from build123d import *

# Parameters (mm, degrees)
SALIENTE_EXTRUIR1_DEPTH = 2
SALIENTE_EXTRUIR2_DEPTH = 2
SALIENTE_EXTRUIR3_DEPTH = 2
CROQUIS5_W              = 22
CROQUIS5_H              = 2
SALIENTE_EXTRUIR4_DEPTH = 17
CROQUIS6_W              = 26
CROQUIS6_H              = 2
SALIENTE_EXTRUIR5_DEPTH = 3
CROQUIS7_W              = 9.109165418
CROQUIS7_H              = 2
CROQUIS7_W_2            = 9.958756631
SALIENTE_EXTRUIR6_DEPTH = 20
CHAFL_N1_SIZE           = 1
CHAFL_N2_SIZE           = 1
CHAFL_N2_SIZE_2         = 0.713515305
CROQUIS8_R              = 8
SALIENTE_EXTRUIR7_DEPTH = 9


with BuildPart() as part:
    # Croquis1 → Saliente-Extruir1 (new body)
    with BuildSketch(Plane.XY):
        Polygon((-2, 23.6), (-2, 20.4), (-2, -5.284781413), (24, -5.284781413), (24, 20.4), (24, 23.6), align=None)
    extrude(amount=SALIENTE_EXTRUIR1_DEPTH)

    # Croquis2 → Saliente-Extruir2 (add)
    with BuildSketch(Plane(origin=(24, 0, 0), x_dir=(0, 0, -1), z_dir=(1, 0, 0))):
        Polygon((0, 23.6), (37.896029649, 23.6), (0, -5.284781413), align=None)
    extrude(amount=-SALIENTE_EXTRUIR2_DEPTH)

    # Croquis4 → Saliente-Extruir3 (add)
    with BuildSketch(Plane.ZY.offset(2)):
        with BuildLine():
            Line((-37.896029649, 23.6), (0, 23.6))
            Line((0, 23.6), (0, -5.284781413))
            Line((0, -5.284781413), (-9.534216457, 1.982305954))
            ThreePointArc((-9.534216457, 1.982305954), (-4.573867025, 12.209468647), (-13.454047634, 19.304700538))
            Line((-13.454047634, 19.304700538), (-32.260716249, 19.304700538))
            Line((-32.260716249, 19.304700538), (-37.896029649, 23.6))
        make_face()
    extrude(amount=-SALIENTE_EXTRUIR3_DEPTH)

    # Croquis5 → Saliente-Extruir4 (add)
    with BuildSketch(Plane(origin=(0, 0, 0), x_dir=(-1, 0, 0), z_dir=(0, 0, -1))):
        with Locations((-11, 22.6)):
            Rectangle(CROQUIS5_W, CROQUIS5_H)
    extrude(amount=SALIENTE_EXTRUIR4_DEPTH)

    # Croquis6 → Saliente-Extruir5 (add)
    with BuildSketch(Plane(origin=(0, 0, 0), x_dir=(-1, 0, 0), z_dir=(0, 0, -1))):
        with Locations((-11, -4.284781413)):
            Rectangle(CROQUIS6_W, CROQUIS6_H)
    extrude(amount=SALIENTE_EXTRUIR5_DEPTH)

    # Croquis7 → Saliente-Extruir6 (add)
    with BuildSketch(Plane(origin=(0, 0, -17), x_dir=(-1, 0, 0), z_dir=(0, 0, -1))):
        with Locations((-4.554582709, 22.6)):
            Rectangle(CROQUIS7_W, CROQUIS7_H)
        with Locations((-17.020621685, 22.6)):
            Rectangle(CROQUIS7_W_2, CROQUIS7_H)
    extrude(amount=SALIENTE_EXTRUIR6_DEPTH)

    # Chaflán1
    chafl_n1_edges = [part.edges().sort_by_distance(p)[0] for p in [
        (17.020621684, 21.6, -37),
        (4.554582709, 21.6, -37),
    ]]
    chamfer(chafl_n1_edges, length=CHAFL_N1_SIZE)

    # Chaflán2
    # the kernel refuses this chamfer: 1, 0.713515305 mm, written as the material it takes off along each edge
    with BuildSketch(Plane(origin=(26.571682988, 23.6, -37.896029649), x_dir=(0, 0, 1), z_dir=(-1, 0, 0))) as chafl_n2_piece_1:
        Polygon((CHAFL_N2_SIZE, 0), (CHAFL_N2_SIZE_2 * 0.79531418588, -CHAFL_N2_SIZE_2 * 0.606197446726), (0, 0), align=None)
    extrude(amount=7.143365976, mode=Mode.SUBTRACT)
    # the kernel refuses this chamfer: 1, 0.713515305 mm, written as the material it takes off along each edge
    with BuildSketch(Plane(origin=(22, 23.6, -37), x_dir=(0, 0, 1), z_dir=(-1, 0, 0))) as chafl_n2_2_piece_1_section:
        Polygon((CHAFL_N2_SIZE, 0), (0, -CHAFL_N2_SIZE), (0, 0), align=None)
    chafl_n2_2_piece_1 = extrude(amount=12.530439619, mode=Mode.PRIVATE)
    chafl_n2_2_piece_1 = split(chafl_n2_2_piece_1, bisect_by=Plane(origin=(22, 23.548014824, -36.948014824), z_dir=(-1.533293416683386e-15, 0.7071067811865533, -0.7071067811865418)), keep=Keep.TOP, mode=Mode.PRIVATE)
    add(chafl_n2_2_piece_1, mode=Mode.SUBTRACT)
    # the kernel refuses this chamfer: 1, 0.713515305 mm, written as the material it takes off along each edge
    with BuildSketch(Plane(origin=(-4.571682988, 23.6, -37.896029649), x_dir=(0, -0.6061974471264424, 0.7953141864052119), z_dir=(1, 0, 0))) as chafl_n2_3_piece_1:
        Polygon((CHAFL_N2_SIZE, 0), (CHAFL_N2_SIZE_2 * 0.79531418588, -CHAFL_N2_SIZE_2 * 0.606197446726), (0, 0), align=None)
    extrude(amount=7.143365976, mode=Mode.SUBTRACT)

    # Croquis8 → Saliente-Extruir7 (add)
    with BuildSketch(Plane.XY.offset(2)):
        with Locations((11, 9.157609293)):
            Circle(CROQUIS8_R)
    extrude(amount=SALIENTE_EXTRUIR7_DEPTH)


solid = part.part
Read the model definition and answer for the solid it produces. Units are mm, in the model's axes. A direction names the side the tool comes from. Give positions to 0.01 mm unless a question says otherwise; leave off trailing zeros. Write each loop counter-clockwise with the first axis right and the second up, starting at its lowest first coordinate (ties: lowest second). Pieces come first, ordered by that corner, then holes. Notation, with made-up numbers: (-22, 82) -> (37, 82) arc R15 cw to (37, 93) -> close; hole circle Ø10 at (53, 38). An arc over 180 degrees is marked (long way). Answer as a JSON object with one key per item and string values. Group by question number.
1) Each of these flat-tipped pins is pushed along its axis until it touches: P1, Ø8, axis at x = 12.5, y = 1.5, coming from the -Z side; P2, Ø1.6, axis at x = 9.5, y = -4, coming from the -Z side; P3, Ø1, axis at x = 15, y = 23, coming from the -Z side. Where does it stop, or does it pass through?
2) Consider L1, parallel to X at y = 6.5, z = -1.5; L2, parallel to Z at x = 10, y = 2; L3, parallel to Z at x = 19.5, y = 13. Determine where each line is inside the solid, lowest interval first. Write a range as from..to.
3) Find section B-B (z = -27). Write down the section's boundary in (x, y).
4) Find section C-C (y = -1.25). Write down the section's boundary in (x, z), and give its area (3 significant figures).
5) Find section D-D (z = -19.5). Write down the section's boundary in (x, y).
6) Find section A-A (x = 11). Write down the section's boundary in (y, z), and give its area (3 significant figures).
7) The mould has two halves that part along X. Classify faces 1 (the flat face through (11, -3.285, -1)), 2 (the flat face through (5, 3, 2)), 3 (the flat face through (11, 23, -17)), 4 (the flat face through (24, 12, -13)): +X half, -X half, draft (parallel to the pull), parting line (faces both ways), or undercut.
8) A tool of negligible diameter and unlimited length cuts with its end or side. For faces 5 (the cylindrical face through (-1.014, 12.042, -4.538)), 6 (the flat face through (11, -4, -3)), 7 (the flat face through (22, 12, -14)), 8 (the flat face through (9.109, 23, -27)), 9 (the flat face through (-1, 19.305, -23)), from which of +Z, -Z, +X, -X, +Y, -Y can it reach the whole face along a straight path? Write none if from no direction.
Values follow:
{
 "1": {"P1": "stops at z = 0", "P2": "stops at z = -3", "P3": "stops at z = -37"},
 "2": {"L1": "x = -2..0, 22..24", "L2": "z = 0..11", "L3": "z = 0..2"},
 "3": {"outline": "(-2, 19.3) -> (0, 19.3) -> (0, 21.6) -> (9.11, 21.6) -> (9.11, 23.6) -> (-2, 23.6) -> close; (12.04, 21.6) -> (22, 21.6) -> (22, 15.29) -> (24, 15.29) -> (24, 23.6) -> (12.04, 23.6) -> close"},
 "4": {"outline": "(-2, -5.29) -> (0, -5.29) -> (0, 0) -> (22, 0) -> (22, -5.29) -> (24, -5.29) -> (24, 2) -> (-2, 2) -> close", "area": "73.2 mm2"},
 "5": {"outline": "(-2, 19.3) -> (0, 19.3) -> (0, 21.6) -> (9.11, 21.6) -> (9.11, 23.6) -> (-2, 23.6) -> close; (12.04, 21.6) -> (22, 21.6) -> (22, 9.58) -> (24, 9.58) -> (24, 23.6) -> (12.04, 23.6) -> close"},
 "6": {"outline": "(-5.28, -3) -> (-3.28, -3) -> (-3.28, 0) -> (21.6, 0) -> (21.6, -17) -> (23.6, -17) -> (23.6, 2) -> (17.16, 2) -> (17.16, 11) -> (1.16, 11) -> (1.16, 2) -> (-5.28, 2) -> close", "area": "242 mm2"},
 "7": {"face 1": "undercut", "face 2": "draft", "face 3": "undercut", "face 4": "+X half"},
 "8": {"face 5": "-Z, -X", "face 6": "-Z, +X, -X, -Y", "face 7": "-Z", "face 8": "-Z, +Y, -Y", "face 9": "-Z, -X, -Y"}
}
